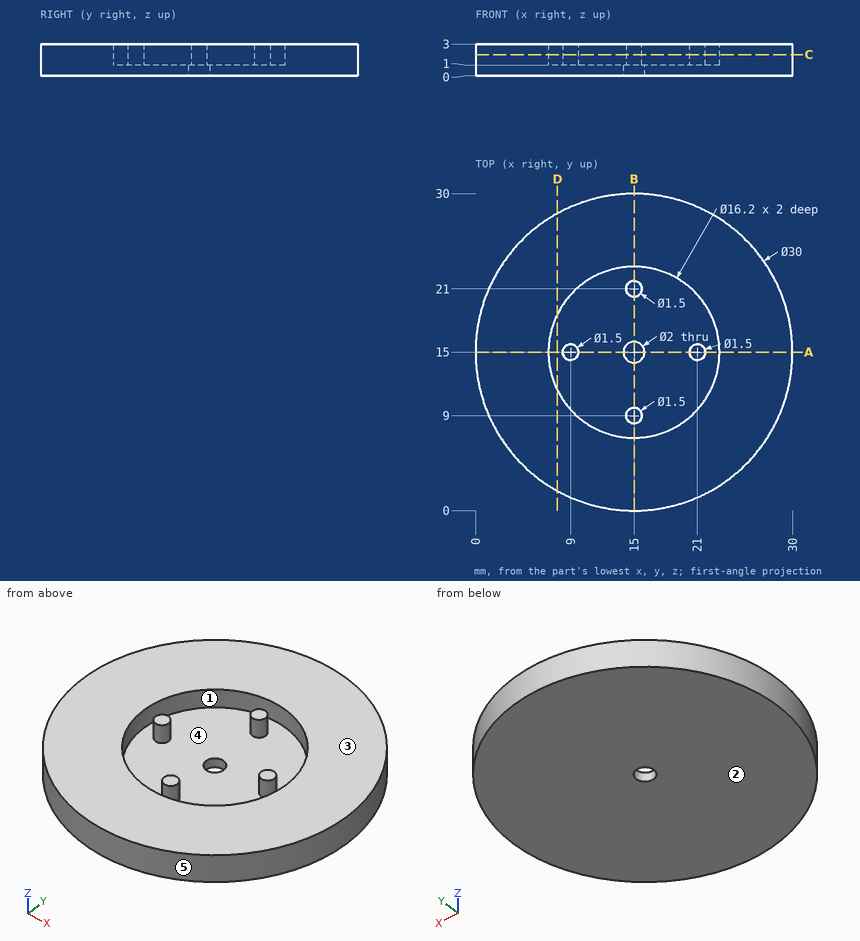
Here's the drawing with two shaded views (mm, measured from the low corner). I have some questions. A direction names the side the tool comes from. Give positions to 0.01 mm unless a question says otherwise; leave off trailing zeros. Loops run counter-clockwise (first coordinate to the right, second up) from the corner with the lowest first, then second, coordinate; pieces in that order, holes last. Notation, with made-up numbers: (28.25, 69.25) - (51.25, 69.25) arc R22 cw to (51.25, 97.25) - close; hole circle Ø10 at (79.25, 18.5). An arc over 180 degrees is marked (long way). Return JSON: item names as keys, results as strings.
1. I'm going to push a flat-ended pin straight in: pin 1 Ø1.5 at (x, z) = (19.5, 0.5) entering from +Y. Where does the tip first touch, or does it pass through?
Output values:
{"pin 1": "stops at y = 29.52"}
2. I want a section at D-D on x = 7.75. Please give me the cut outline in (y, z).
Output values:
{"outline": "(1.87, 0) - (28.13, 0) - (28.13, 3) - (18.61, 3) - (18.61, 1) - (11.39, 1) - (11.39, 3) - (1.87, 3) - close"}
3. For the marked faces 1 and 2, which set-ups out of +Z, -Z, +X, -X, +Y, -Y let a thin tool reach every point of the face, with its end or its side?
Output values:
{"face 1": "+Z", "face 2": "-Z, +X, -X, +Y, -Y"}
4. We'd pull the mould along X, two halves only. Please class the marked faces 3, 4 and 5: +X half, -X half, draft (parallel to the pull), parting line (faces both ways), or undercut.
Output values:
{"face 3": "draft", "face 4": "undercut", "face 5": "parting line"}
5. I want a section at C-C on z = 2. Please give me the cut outline in (x, y).
Output values:
{"outline": "circle Ø30 at (15, 15); circle Ø1.5 at (9, 15); circle Ø1.5 at (15, 9); circle Ø1.5 at (15, 21); circle Ø1.5 at (21, 15); hole circle Ø16.2 at (15, 15)"}
6. I want a section at A-A on y = 15. Please give me the cut outline in (x, z).
Output values:
{"outline": "(0, 0) - (14, 0) - (14, 1) - (9.75, 1) - (9.75, 3) - (8.25, 3) - (8.25, 1) - (6.9, 1) - (6.9, 3) - (0, 3) - close; (16, 0) - (30, 0) - (30, 3) - (23.1, 3) - (23.1, 1) - (21.75, 1) - (21.75, 3) - (20.25, 3) - (20.25, 1) - (16, 1) - close"}
7. If I drill on line 1 (Y direction, x = 15, z = 2.25); line 2 (X direction, y = 15.5, z = 1.8), over which ranges is the centre line in solid material (lowest first)?
Output values:
{"line 1": "y = 0 to 6.9, 8.25 to 9.75, 20.25 to 21.75, 23.1 to 30", "line 2": "x = 0.01 to 6.92, 8.44 to 9.56, 20.44 to 21.56, 23.08 to 29.99"}
